```python
from build123d import *

# Parameters (mm, degrees)
SKETCH1_R               = 5
BOSS_EXTRUDE1_DEPTH     = 10
SKETCH2_W               = 80
SKETCH2_H               = 5
BOSS_EXTRUDE2_DEPTH     = 50
SKETCH3_W               = 5
SKETCH3_H               = 50
BOSS_EXTRUDE3_DEPTH     = 16
FILLET1_R               = 50
FILLET3_R               = 5
FILLET7_R               = 5
FILLET8_R               = 5
CUT_EXTRUDE4_DEPTH      = 32
CUT_EXTRUDE4_DEPTH_BACK = 2
SKETCH8_W               = 5
SKETCH8_H               = 50
SKETCH11_R              = 10
BOSS_EXTRUDE5_DEPTH     = 18.75
CUT_EXTRUDE9_DEPTH      = 45


with BuildPart() as part:
    # Sketch1 → Boss-Extrude1 (new body)
    with BuildSketch(Plane.XY):
        with BuildLine():
            Line((-40, 5), (-40, 0))
            Line((-40, 0), (40, 0))
            Line((40, 0), (40, 5))
            Line((40, 5), (35, 5))
            Line((35, 5), (35, 75))
            Line((35, 75), (9.645273695, 167.639828659))
            ThreePointArc((9.645273695, 167.639828659), (0, 175), (-9.645273695, 167.639828659))
            Line((-9.645273695, 167.639828659), (-35, 75))
            Line((-35, 75), (-35, 5))
            Line((-35, 5), (-40, 5))
        make_face()
        with Locations((0, 165)):
            Circle(SKETCH1_R, mode=Mode.SUBTRACT)
    extrude(amount=BOSS_EXTRUDE1_DEPTH)

    # Sketch2 → Boss-Extrude2 (add)
    with BuildSketch(Plane(origin=(0, 0, 0), x_dir=(-1, 0, 0), z_dir=(0, 0, -1))):
        with Locations((0, 2.5)):
            Rectangle(SKETCH2_W, SKETCH2_H)
    extrude(amount=BOSS_EXTRUDE2_DEPTH)

    # Sketch3 → Boss-Extrude3 (add)
    with BuildSketch(Plane(origin=(0, 0, 0), x_dir=(-1, 0, 0), z_dir=(0, 0, -1))):
        with Locations((-17.5, 75)):
            Rectangle(SKETCH3_W, SKETCH3_H)
        with Locations((17.5, 75)):
            Rectangle(SKETCH3_W, SKETCH3_H)
    extrude(amount=BOSS_EXTRUDE3_DEPTH)

    # Fillet1
    fillet1_edges = [part.edges().sort_by_distance(p)[0] for p in [
        (-35, 75, 5),
        (35, 75, 5),
    ]]
    fillet(fillet1_edges, radius=FILLET1_R)

    # Fillet3
    fillet3_edges = [part.edges().sort_by_distance(p)[0] for p in [
        (0, 5, -50),
        (-40, 5, -20),
        (40, 5, -20),
    ]]
    fillet(fillet3_edges, radius=FILLET3_R - 0.0001)  # a hair under: the kernel refuses the full size

    # Fillet7
    fillet7_edges = [part.edges().sort_by_distance(p)[0] for p in [
        (20, 75, -16),
        (20, 50, -8),
        (20, 100, -8),
    ]]
    fillet(fillet7_edges, radius=FILLET7_R - 0.0001)  # a hair under: the kernel refuses the full size

    # Fillet8
    fillet8_edges = [part.edges().sort_by_distance(p)[0] for p in [
        (-20, 50, -8),
        (-20, 75, -16),
        (-20, 100, -8),
    ]]
    fillet(fillet8_edges, radius=FILLET8_R - 0.0001)  # a hair under: the kernel refuses the full size

    # Sketch8 → Cut-Extrude4 (cut, two sides: drawn at the far end of the back side and taken through both)
    with BuildSketch(Plane(origin=(-15, 0, 0), x_dir=(0, 0, -1), z_dir=(1, 0, 0)).offset(-CUT_EXTRUDE4_DEPTH_BACK)):
        with Locations((8.5, 75)):
            Rectangle(SKETCH8_W, SKETCH8_H)
    extrude(amount=CUT_EXTRUDE4_DEPTH + CUT_EXTRUDE4_DEPTH_BACK, mode=Mode.SUBTRACT)

    # Sketch11 → Boss-Extrude5 (add)
    with BuildSketch(Plane(origin=(0, 5, 0), x_dir=(1, 0, 0), z_dir=(0, 1, 0))):
        with Locations(Location((0, 16.5, 0), (0, 0, 90))):
            Circle(SKETCH11_R)
    extrude(amount=BOSS_EXTRUDE5_DEPTH)

    # Sketch14 → Cut-Extrude9 (cut)
    with BuildSketch(Plane(origin=(0, 0, 0), x_dir=(-1, 0, 0), z_dir=(0, 0, -1))):
        with BuildLine():
            Line((-25, 35), (-25, 20))
            ThreePointArc((-25, 20), (-23.535533906, 16.464466094), (-20, 15))
            Line((-20, 15), (20, 15))
            ThreePointArc((20, 15), (23.535533906, 16.464466094), (25, 20))
            Line((25, 20), (25, 35))
            ThreePointArc((25, 35), (23.535533906, 38.535533906), (20, 40))
            Line((20, 40), (-20, 40))
            ThreePointArc((-20, 40), (-23.535533906, 38.535533906), (-25, 35))
        make_face()
        with BuildLine():
            ThreePointArc((-3.959742989, 150.532089458), (0, 150), (3.959742989, 150.532089458))
            Line((3.959742989, 150.532089458), (15.05302813, 110))
            Line((15.05302813, 110), (-15.05302813, 110))
            Line((-15.05302813, 110), (-3.959742989, 150.532089458))
        make_face()
        with BuildLine():
            Line((-10, 95), (-10, 55))
            ThreePointArc((-10, 55), (-8.535533906, 51.464466094), (-5, 50))
            Line((-5, 50), (5, 50))
            ThreePointArc((5, 50), (8.535533906, 51.464466094), (10, 55))
            Line((10, 55), (10, 95))
            ThreePointArc((10, 95), (8.535533906, 98.535533906), (5, 100))
            Line((5, 100), (-5, 100))
            ThreePointArc((-5, 100), (-8.535533906, 98.535533906), (-10, 95))
        make_face()
    extrude(amount=-CUT_EXTRUDE9_DEPTH, mode=Mode.SUBTRACT)


solid = part.part
```
The model under review builds one solid part; all positions refer to its coordinate system, in mm. A direction names the side the tool comes from. Give positions to 0.01 mm unless a question says otherwise; leave off trailing zeros. Answer in a Markdown table with one row per item.
Item 1: For P1, Ø3.5, axis at y = 75, z = -4, coming from the -X side; P2, Ø5, axis at x = 31.5, y = 52.5, coming from the -Z side; P3, Ø16, axis at x = -3.5, z = -14, coming from the +Y side, all flat-tipped, find the tip position at first contact; note any pin that passes through.
Check sheet entries:
| item | result |
|---|---|
| P1 | x = -20 |
| P2 | z = 0 |
| P3 | y = 23.75 |
Item 2: Add section A-A on x = 0. State how many separate pieces and enclosed holes the cut face has, plus the area to 3 significant figures.
Check sheet entries:
| item | result |
|---|---|
| separate pieces | 5 |
| enclosed holes | 0 |
| area | 1,120 mm2 |
Item 3: Tool access review of faces 4 (the face through (-17, 75, -8)), 5 (the face through (-15, 75, -13)), 6 (the face through (-10, 75, 5)), 7 (the face through (-19, 75, -14)), 8 (the face through (35, 36, 5)): name each direction out of +Z, -Z, +X, -X, +Y, -Y from which nothing blocks a thin tool from reaching the whole face with its end or side.
Check sheet entries:
| item | result |
|---|---|
| face 4 | +Y |
| face 5 | -Z, +Y |
| face 6 | +Z, -Z |
| face 7 | -Z, -X, +Y |
| face 8 | +Z, -Z, +X, +Y |
Item 4: Draft analysis for pull direction Y (two halves, no side actions). For faces 1 (the face through (20, 75, -5)), 2 (the face through (-18, 99, -6)), 3 (the face through (-23, 16, 5)), state which applies: +Y half, -Y half, draft (parallel to the pull), parting line (faces both ways), or undercut.
Check sheet entries:
| item | result |
|---|---|
| face 1 | draft |
| face 2 | +Y half |
| face 3 | undercut |
Item 5: For line 1 along Y through (x, z) = (0, 2.5); line 2 along Z through (x, y) = (-15, 103); line 3 along Y through (x, z) = (-2, -24.5), list the stretches that pass through material, from the lowest coordinate up.
Check sheet entries:
| item | result |
|---|---|
| line 1 | 0 to 15, 40 to 50, 100 to 110, 150 to 160, 170 to 175 |
| line 2 | 0 to 10 |
| line 3 | 0 to 23.75 |
